from build123d import *

# Parameters (mm, degrees)
CHAMFER_1_SIZE      = 1.374
SKETCH_2_W          = 22
SKETCH_2_H          = 5
CUT_EXTRUDE_1_DEPTH = 15


with BuildPart() as part:
    # Эскиз1 → Повернуть1 (revolve)
    with BuildSketch(Plane.XY, mode=Mode.PRIVATE) as revolve_1_sk:
        Polygon((0, 0), (299, 0), (299, 10), (274, 10), (274, 9), (272, 9), (272, 15), (60, 15), (60, 12), (25, 12), (25, 10), (0, 10), align=None)
    revolve(revolve_1_sk.sketch.rotate(Axis((-1007.978642663, 0, 0), (1, 0, 0)), 90), axis=Axis((-1007.978642663, 0, 0), (1, 0, 0)))

    # Фаска1
    chamfer_1_edges = [part.edges().sort_by_distance(p)[0] for p in [
        (0, 0, -10),
        (299, 0, -10),
    ]]
    chamfer(chamfer_1_edges, length=CHAMFER_1_SIZE)

    # Эскиз2 → Вырез-Вытянуть1 (cut, symmetric)
    with BuildSketch(Plane(origin=(0, 0, 0), x_dir=(1, 0, 0), z_dir=(0, 1, 0))):
        with Locations((263, 12.5)):
            Rectangle(SKETCH_2_W, SKETCH_2_H)
        with Locations((263, -12.5)):
            Rectangle(SKETCH_2_W, SKETCH_2_H)
    extrude(amount=CUT_EXTRUDE_1_DEPTH, both=True, mode=Mode.SUBTRACT)


solid = part.part
Could you check a few things on this model? Use its own coordinates, in mm. A direction names the side the tool comes from. Coordinates: 2 decimals unless noted, no trailing zeros. Write each loop counter-clockwise with the first axis right and the second up, starting at its lowest first coordinate (ties: lowest second). Pieces come first, ordered by that corner, then holes. Notation, with made-up numbers: (59.25, 38.5) - (91.25, 38.5) arc R19 cw to (91.25, 67.5) - close; hole circle Ø6 at (16.25, 30.5). An arc over 180 degrees is marked (long way). Put each result on its own line as item: value. Start each with the question number.
Q1. Which directions (+Z, -Z, +X, -X, +Y, -Y) give clear straight access to the entire face, cutting with the end or side of a thin tool? Please do faces 1 (the cylindrical face through (286, 0, -10)), 2 (the cylindrical face through (42.255, -3.604, 11.446)), 3 (the flat face through (262, 0, 10)).
Q2. I want a section at D-D on x = 106. Write out the boundary of the cut face in (y, z), plus the area to 3 significant figures.
Q3. Please list where these lines run through material, in increasing order: L1, parallel to X at y = -6.75, z = -9.25; L2, parallel to Z at x = 115, y = -10; L3, parallel to Y at x = 14, z = 1.
Q4. I'm going to push flat-ended pins straight in: P1, Ø10, axis at x = 258, y = -5, coming from the +Z side; P2, Ø1.5, axis at x = 123.5, y = -10, coming from the -Z side; P3, Ø8, axis at x = 94.5, z = -10, coming from the -Y side; P4, Ø6, axis at y = 3, z = 10, coming from the +X side. Where does each tip first touch, or does it pass through?
Q5. I want a section at A-A on z = 0. Write out the boundary of the cut face in (x, y), plus the area to 3 significant figures.
Q6. Thinking about a two-plate mould opening in X: for faces 4 (the cylindrical face through (272.986, -6.083, -6.633)), 5 (the flat face through (0, 0, 0)), 6 (the flat face through (252, 0, 12)), which applies, pulls with the +X half, pulls with the -X half, needs draft (parallel to the pull), parting line crosses it, or undercut?
Q7. I want a section at B-B on y = 0. Write out the boundary of the cut face in (x, z), plus the area to 3 significant figures.
Q8. I want a section at C-C on x = 267. Write out the boundary of the cut face in (y, z).
Checks:
1. face 1: +X
1. face 2: -X
1. face 3: +Z, +X, +Y, -Y
2. outline: circle Ø30 at (0, 0)
2. area: 707 mm²
3. L1: 25 to 272
3. L2: -11.18 to 11.18
3. L3: -9.95 to 9.95
4. P1: z = 10
4. P2: z = -11.81
4. P3: y = -13.75
4. P4: x = 299
5. outline: (0, -8.63) - (1.37, -10) - (25, -10) - (25, -12) - (60, -12) - (60, -15) - (272, -15) - (272, -9) - (274, -9) - (274, -10) - (297.63, -10) - (299, -8.63) - (299, 8.63) - (297.63, 10) - (274, 10) - (274, 9) - (272, 9) - (272, 15) - (60, 15) - (60, 12) - (25, 12) - (25, 10) - (1.37, 10) - (0, 8.63) - close
5. area: 8,230 mm²
6. face 4: undercut
6. face 5: pulls with the -X half
6. face 6: pulls with the +X half
7. outline: (0, -8.63) - (1.37, -10) - (25, -10) - (25, -12) - (60, -12) - (60, -15) - (252, -15) - (252, -10) - (272, -10) - (272, -9) - (274, -9) - (274, -10) - (297.63, -10) - (299, -8.63) - (299, 8.63) - (297.63, 10) - (274, 10) - (274, 9) - (272, 9) - (272, 10) - (252, 10) - (252, 15) - (60, 15) - (60, 12) - (25, 12) - (25, 10) - (1.37, 10) - (0, 8.63) - close
7. area: 8,030 mm²
8. outline: (-11.18, -10) - (11.18, -10) arc R15 ccw to (11.18, 10) - (-11.18, 10) arc R15 ccw to start
